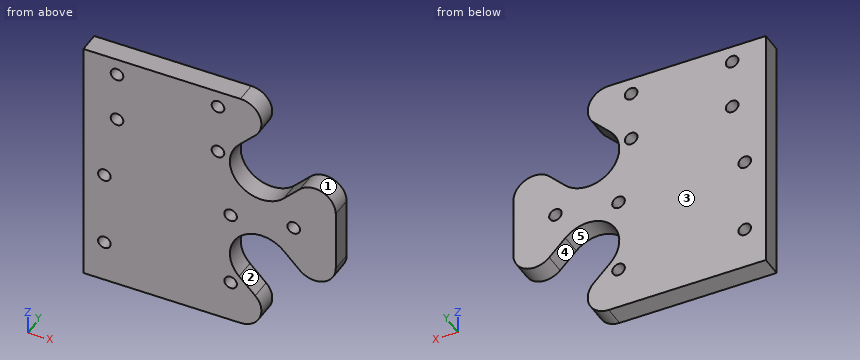
from build123d import *

# Parameters (mm, degrees)
SKETCH_1_W          = 60
SKETCH_1_H          = 60
EXTRUDE_1_DEPTH     = 5
CUT_EXTRUDE_1_DEPTH = 43.720018727
FILLET_1_R          = 5
SKETCH_3_R          = 1.5
CUT_EXTRUDE_2_DEPTH = 43.720018727


with BuildPart() as part:
    # 草图1 → 凸台-拉伸1 (new body)
    with BuildSketch(Plane(origin=(0, 0, 0), x_dir=(1, 0, 0), z_dir=(0, 1, 0))):
        Rectangle(SKETCH_1_W, SKETCH_1_H)
    extrude(amount=EXTRUDE_1_DEPTH)

    # 草图2 → 切除-拉伸1 (cut, through all)
    with BuildSketch(Plane(origin=(0, 5, 0), x_dir=(1, 0, 0), z_dir=(0, 1, 0))):
        with BuildLine():
            Line((19.393398282, 30), (7.019029611, 17.625631329))
            ThreePointArc((7.019029611, 17.625631329), (7.019029611, 7.019029611), (17.625631329, 7.019029611))
            Line((17.625631329, 7.019029611), (30, 19.393398282))
            Line((30, 19.393398282), (30, 30))
            Line((30, 30), (19.393398282, 30))
        make_face()
        with BuildLine():
            Line((19.393398282, -30), (30, -30))
            Line((30, -30), (30, -19.393398282))
            Line((30, -19.393398282), (17.625631329, -7.019029611))
            ThreePointArc((17.625631329, -7.019029611), (7.019029611, -7.019029611), (7.019029611, -17.625631329))
            Line((7.019029611, -17.625631329), (19.393398282, -30))
        make_face()
    extrude(amount=-CUT_EXTRUDE_1_DEPTH, mode=Mode.SUBTRACT)

    # 圆角1
    fillet_1_edges = [part.edges().sort_by_distance(p)[0] for p in [
        (30, 2.5, -19.393398282),
        (19.393398282, 2.5, -30),
        (19.393398282, 2.5, 30),
        (30, 2.5, 19.393398282),
    ]]
    fillet(fillet_1_edges, radius=FILLET_1_R)

    # 草图3 → 切除-拉伸2 (cut, through all)
    with BuildSketch(Plane(origin=(0, 5, 0), x_dir=(1, 0, 0), z_dir=(0, 1, 0))):
        with Locations(Location((20, 0, 0), (0, 0, 270))):
            Circle(SKETCH_3_R)
        with Locations(Location((-22, -14, 0), (0, 0, 270))):
            Circle(SKETCH_3_R)
        with Locations(Location((2, -14, 0), (0, 0, 90))):
            Circle(SKETCH_3_R)
        with Locations(Location((2, -26, 0), (0, 0, 270))):
            Circle(SKETCH_3_R)
        with Locations(Location((-22, -26, 0), (0, 0, 90))):
            Circle(SKETCH_3_R)
        with Locations(Location((-25, 20, 0), (0, 0, 270))):
            Circle(SKETCH_3_R)
        with Locations(Location((5, 20, 0), (0, 0, 90))):
            Circle(SKETCH_3_R)
        with Locations(Location((-25, 2, 0), (0, 0, 270))):
            Circle(SKETCH_3_R)
        with Locations(Location((5, 2, 0), (0, 0, 270))):
            Circle(SKETCH_3_R)
    extrude(amount=-CUT_EXTRUDE_2_DEPTH, mode=Mode.SUBTRACT)


solid = part.part
Work out the finished part from the listing and answer in its coordinate system (mm). Face numbers are marked on the shaded views. A direction names the side the tool comes from. Round coordinates to 2 decimals unless told otherwise and drop trailing zeros. Write each loop counter-clockwise with the first axis right and the second up, starting at its lowest first coordinate (ties: lowest second). Pieces come first, ordered by that corner, then holes. Notation, with made-up numbers: (65, 13) - (99, 13) arc R16 cw to (99, 32) - close; hole circle Ø10 at (87, -31.75). An arc over 180 degrees is marked (long way). Answer in a Markdown table with one row per item. Add a question column.
1. A cutting plane is placed at C-C, the plane z = 14. Determine the outline of the cut face in (x, y).
2. A cutting plane is placed at A-A, the plane x = -22. Determine the outline of the cut face in (y, z), and give its area (3 significant figures).
3. A cutting plane is placed at B-B, the plane y = 1. Count the separate pieces of the cut face and the enclosed holes in it, and give its area (3 significant figures).
4. The mould has two halves that part along X. Classify the marked faces 1, 2 and 3: +X half, -X half, draft (parallel to the pull), parting line (faces both ways), or undercut.
5. Find the intervals of material crossed by line 1 along X through (y, z) = (2.65, 14); line 2 along X through (y, z) = (1.1, -2); line 3 along X through (y, z) = (0.85, -8.5), in increasing order. Write a range as from..to.
6. For the marked faces 4 and 5, determine the directions among +Z, -Z, +X, -X, +Y, -Y from which every point of the face is accessible in a straight line to the end or side of a thin tool.
7. A cutting plane is placed at D-D, the plane x = 20. Determine the outline of the cut face in (y, z).
8. Given pin 1 (1.5 mm diameter, centred on x = 9.5, y = 2.5, fed in from +Z); pin 2 (1.8 mm diameter, centred on x = -22, z = 26, fed in from +Y), each flat-ended and moving along its own axis, determine where each tip first touches the part or whether it passes through.
Worked out:
| question | item | result |
|---|---|---|
| 1 | outline | (-30, 0) - (-23.5, 0) - (-23.5, 5) - (-30, 5) - close; (-20.5, 0) - (0.5, 0) - (0.5, 5) - (-20.5, 5) - close; (3.5, 0) - (5.01, 0) - (5.01, 5) - (3.5, 5) - close |
| 2 | outline | (0, -30) - (5, -30) - (5, 12.5) - (0, 12.5) - close; (0, 15.5) - (5, 15.5) - (5, 24.5) - (0, 24.5) - close; (0, 27.5) - (5, 27.5) - (5, 30) - (0, 30) - close |
| 2 | area | 270 mm^2 |
| 3 | separate pieces | 1 |
| 3 | enclosed holes | 9 |
| 3 | area | 2,600 mm^2 |
| 4 | face 1 | undercut |
| 4 | face 2 | +X half |
| 4 | face 3 | draft |
| 5 | line 1 | -30..-23.5, -20.5..0.5, 3.5..5.01 |
| 5 | line 2 | -30..-26.5, -23.5..3.5, 6.5..30 |
| 5 | line 3 | -30..5.87, 19.11..29.86 |
| 6 | face 4 | -Z, +Y, -Y |
| 6 | face 5 | +Y, -Y |
| 7 | outline | (0, -9.39) - (5, -9.39) - (5, -1.5) - (0, -1.5) - close; (0, 1.5) - (5, 1.5) - (5, 9.39) - (0, 9.39) - close |
| 8 | pin 1 | z = 29.79 |
| 8 | pin 2 | through |
